Geometry: see drawing. Coordinates: mm, zero at the bounding-box minimum. Round coordinates to 2 decimals unless told otherwise and drop trailing zeros. Write each loop counter-clockwise with the first axis right and the second up, starting at its lowest first coordinate (ties: lowest second). Pieces come first, ordered by that corner, then holes.
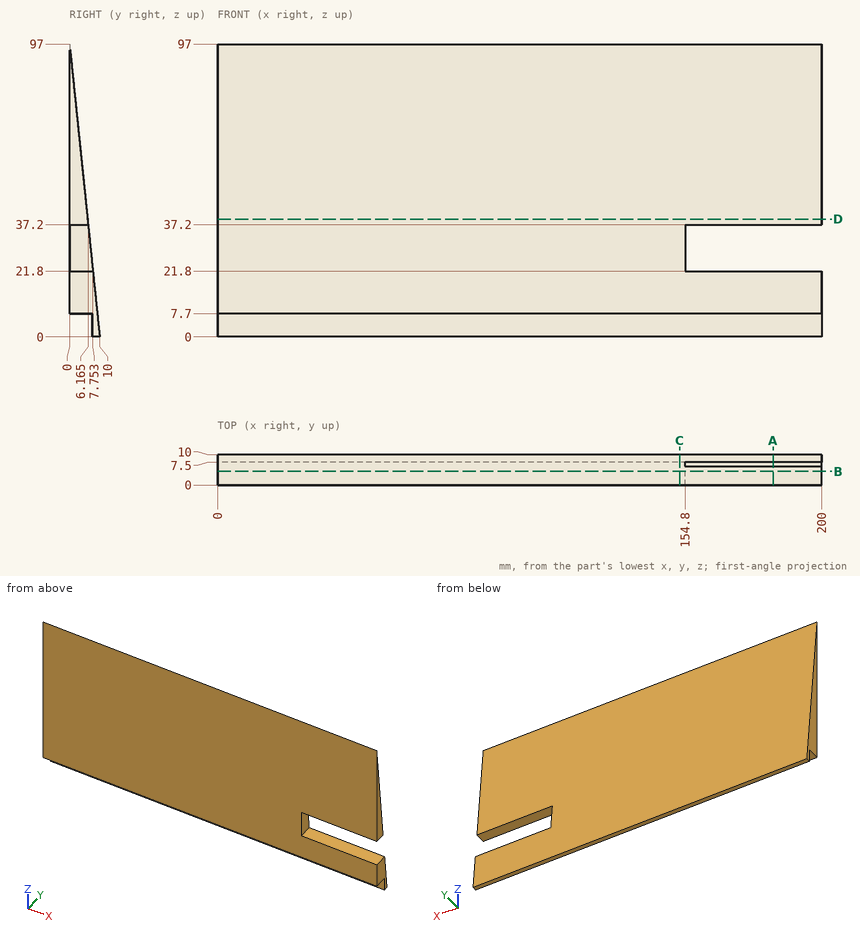
1) Material intervals for line 1 (Y direction, x = 24.5, z = 22.5); line 2 (Y direction, x = 99.5, z = 67); line 3 (X direction, y = 7.25, z = 25), sorted ascending.
Taken from the geometry:
line 1: y = 0 to 7.68
line 2: y = 0 to 3.09
line 3: x = 0 to 154.8
2) Section query D-D on z = 39. Return the cut outline in (x, y), then the cut area to 3 significant figures.
Taken from the geometry:
outline: (0, 0) - (200, 0) - (200, 5.98) - (0, 5.98) - close
area: 1,200 mm2
3) Contact query for flat-ended pins moving along their axis: P1, Ø4, axis at x = 73, z = 53.5, coming from the +Y side; P2, Ø3, axis at x = 186, y = 1.5, coming from the -Z side; P3, Ø6, axis at x = 121, z = 56, coming from the +Y side. Output: stop coordinate, or through.
Taken from the geometry:
P1: stops at y = 4.69
P2: stops at z = 7.7
P3: stops at y = 4.54
4) Section query C-C on x = 153. Return the cut outline in (y, z), then the cut area to 3 significant figures.
Taken from the geometry:
outline: (0, 7.7) - (7.5, 7.7) - (7.5, 0) - (10, 0) - (0, 97) - close
area: 427 mm2
5) Section query B-B on y = 4.5. Return the cut outline in (x, z).
Taken from the geometry:
outline: (0, 7.7) - (200, 7.7) - (200, 21.8) - (154.8, 21.8) - (154.8, 37.2) - (200, 37.2) - (200, 53.35) - (0, 53.35) - close
6) Section query A-A on x = 184. Return the cut outline in (y, z) (1 decimal).
Taken from the geometry:
outline: (0, 7.7) - (7.5, 7.7) - (7.5, 0) - (10, 0) - (7.8, 21.8) - (0, 21.8) - close; (0, 37.2) - (6.2, 37.2) - (0, 97) - close
